The model under review builds one solid part; all positions refer to its coordinate system, in mm. A direction names the side the tool comes from. Give positions to 0.01 mm unless a question says otherwise; leave off trailing zeros. Order: outer loops, then holes, each group sorted by start corner. A loop starts at its lowest first (then second) coordinate and runs counter-clockwise, first axis right, second up.
```python
from build123d import *

# Parameters (mm, degrees)
F1_DEPTH      = 20
F2_DEPTH      = 15
F4_W          = 3.3256819006
F4_H          = 11.2064601853
F5_DEPTH      = 5.2
F5_DEPTH_BACK = 20
F3_R          = 3.6353661433
F6_DEPTH      = 25
F7_T1_DEPTH   = 11.2064601853
F7_T3_DEPTH   = 3.3256819006
F7_T5_DEPTH   = 3.3256819006
F7_T11_DEPTH  = 8.3256819006
F7_T16_DEPTH  = 16.2064601853
F7_T23_DEPTH  = 16.2064601853
F7_T27_DEPTH  = 8.3256819006
F7_T35_DEPTH  = 8.3256819006
F7_T40_DEPTH  = 16.2064601853
F7_T47_DEPTH  = 16.2064601853
F7_T51_DEPTH  = 8.3256819006
F7_T55_DEPTH  = 21.2064601853


# Not quite as in the source:
# - a fillet or chamfer that OpenCascade refuses, or shapes differently, is made with other operations: its cross-section is extruded or revolved along the edge and cut away or added


with BuildPart() as f1:
    # F0 (on Front) → F1 (new body)
    with BuildSketch(Plane.XZ):
        Polygon((7.3840099636, 4.3827313822), (-0.1035517331, 8.5861059014), (-7.4875616967, 4.2033745192), (-7.3840099636, -4.3827313822), (0.1035517331, -8.5861059014), (7.4875616967, -4.2033745192), align=None)
        Polygon((-2.8867513459, 5), (2.8867513459, 5), (5.7735026919, 0), (2.8867513459, -5), (-2.8867513459, -5), (-5.7735026919, 0), align=None, mode=Mode.SUBTRACT)
    extrude(amount=F1_DEPTH)

    # F0 (on Front) → F2 (join)
    with BuildSketch(Plane.XZ):
        Polygon((5.7735026919, 0), (2.8867513459, 5), (-2.8867513459, 5), (-5.7735026919, 0), (-2.8867513459, -5), (2.8867513459, -5), align=None)
    extrude(amount=F2_DEPTH)

    # F4 (on face) → F5 (join, two sides)
    with BuildSketch(Plane(origin=(-3.7955567149, 0, 6.3947402103), x_dir=(0.8599326743, 0, 0.51040748), z_dir=(-0.51040748, 0, 0.8599326743))) as f5_sk:
        with Locations((0, -5.6032300927)):
            Rectangle(F4_W, F4_H)
    extrude(amount=F5_DEPTH)
    extrude(f5_sk.sketch, amount=-F5_DEPTH_BACK)

    # F3 (on face) → F6 (cut)
    with BuildSketch(Plane.XZ.offset(15)):
        Circle(F3_R)
    extrude(amount=-F6_DEPTH, mode=Mode.SUBTRACT)

    # F7: fillet of radius 2 on 10 edges, made by hand

    # F7_s2 → F7_t1 (join)
    with BuildSketch(Plane.XZ):
        with BuildLine():
            ThreePointArc((-6.9453533288, 4.525198791), (-6.0282146576, 5.7507608695), (-6.2463029403, 7.2658790997))
            Line((-6.2463029403, 7.2658790997), (-5.2254879802, 5.5460137511))
            Line((-5.2254879802, 5.5460137511), (-6.9453533288, 4.525198791))
        make_face()
        with BuildLine():
            ThreePointArc((-0.645760101, 8.2642816296), (-2.1608783312, 8.0461933468), (-3.3864404097, 8.963332018))
            Line((-3.3864404097, 8.963332018), (-2.3656254496, 7.2434666695))
            Line((-2.3656254496, 7.2434666695), (-0.645760101, 8.2642816296))
        make_face()
        with BuildLine():
            ThreePointArc((6.9453533288, -4.525198791), (6.0282146576, -5.7507608695), (6.2463029403, -7.2658790997))
            Line((6.2463029403, -7.2658790997), (5.2254879802, -5.5460137511))
            Line((5.2254879802, -5.5460137511), (6.9453533288, -4.525198791))
        make_face()
        with BuildLine():
            ThreePointArc((0.645760101, -8.2642816296), (2.1608783312, -8.0461933468), (3.3864404097, -8.963332018))
            Line((3.3864404097, -8.963332018), (2.3656254496, -7.2434666695))
            Line((2.3656254496, -7.2434666695), (0.645760101, -8.2642816296))
        make_face()
    extrude(amount=F7_T1_DEPTH)

    # F7_s4 → F7_t3 (join)
    with BuildSketch(Plane(origin=(-1.4299312653, 0, -0.8487264592), x_dir=(0, 1, 0), z_dir=(0.8599326743, 0, 0.51040748))):
        with BuildLine():
            ThreePointArc((-13.2064601853, 7.4363265887), (-11.792246623, 8.0221130263), (-11.2064601853, 9.4363265887))
            Line((-11.2064601853, 9.4363265887), (-11.2064601853, 7.4363265887))
            Line((-11.2064601853, 7.4363265887), (-13.2064601853, 7.4363265887))
        make_face()
    extrude(amount=F7_T3_DEPTH)

    # F7_s6 → F7_t5 (join)
    with BuildSketch(Plane(origin=(1.4299312653, 0, 0.8487264592), x_dir=(0, 1, 0), z_dir=(-0.8599326743, 0, -0.51040748))):
        with BuildLine():
            ThreePointArc((-13.2064601853, 7.4363265887), (-11.792246623, 8.0221130263), (-11.2064601853, 9.4363265887))
            Line((-11.2064601853, 9.4363265887), (-11.2064601853, 7.4363265887))
            Line((-11.2064601853, 7.4363265887), (-13.2064601853, 7.4363265887))
        make_face()
    extrude(amount=F7_T5_DEPTH)


with BuildPart() as f7_tool9:
    # F7_s10 → F7_t11 (new body)
    with BuildSketch(Plane(origin=(-5.7295946368, 0, -3.4007638594), x_dir=(0, 1, 0), z_dir=(0.8599326743, 0, 0.51040748))):
        with BuildLine():
            ThreePointArc((-13.2064601853, 7.4363265887), (-11.792246623, 8.0221130263), (-11.2064601853, 9.4363265887))
            Line((-11.2064601853, 9.4363265887), (-11.2064601853, 7.4363265887))
            Line((-11.2064601853, 7.4363265887), (-13.2064601853, 7.4363265887))
        make_face()
    extrude(amount=F7_T11_DEPTH)

    split(bisect_by=Plane(origin=(-7.4357858302, 0, -0.0896784315), x_dir=(0, 1, 0), z_dir=(0.9999272815, 0, 0.0120595069)), keep=Keep.TOP)

    split(bisect_by=Plane(origin=(-1.4299312653, 0, -0.8487264592), x_dir=(0, 1, 0), z_dir=(-0.8599326743, 0, -0.51040748)), keep=Keep.TOP)


with BuildPart() as f7_tool14:
    # F7_s15 → F7_t16 (new body)
    with BuildSketch(Plane.XZ):
        with BuildLine():
            ThreePointArc((-6.9453533288, 4.525198791), (-6.0282146576, 5.7507608695), (-6.2463029403, 7.2658790997))
            Line((-6.2463029403, 7.2658790997), (-5.2254879802, 5.5460137511))
            Line((-5.2254879802, 5.5460137511), (-6.9453533288, 4.525198791))
        make_face()
    extrude(amount=F7_T16_DEPTH)

    split(bisect_by=Plane.XZ.offset(11.2064601853), keep=Keep.TOP)


with BuildPart() as f7_tool9_1:
    add(f7_tool9.part)

    # F7_t18: intersect F7_tool14
    add(f7_tool14.part, mode=Mode.INTERSECT)


with BuildPart() as f1_1:
    add(f1.part)

    # F7_t7: union F7_tool9
    add(f7_tool9_1.part)


with BuildPart() as f7_tool21:
    # F7_s22 → F7_t23 (new body)
    with BuildSketch(Plane.XZ.offset(16.2064601853)):
        with BuildLine():
            ThreePointArc((-0.645760101, 8.2642816296), (-2.1608783312, 8.0461933468), (-3.3864404097, 8.963332018))
            Line((-3.3864404097, 8.963332018), (-2.3656254496, 7.2434666695))
            Line((-2.3656254496, 7.2434666695), (-0.645760101, 8.2642816296))
        make_face()
    extrude(amount=-F7_T23_DEPTH)

    split(bisect_by=Plane.XZ.offset(11.2064601853), keep=Keep.TOP)


with BuildPart() as f7_tool25:
    # F7_s26 → F7_t27 (new body)
    with BuildSketch(Plane(origin=(-1.4299312653, 0, -0.8487264592), x_dir=(0, 1, 0), z_dir=(0.8599326743, 0, 0.51040748))):
        with BuildLine():
            ThreePointArc((-13.2064601853, 7.4363265887), (-11.792246623, 8.0221130263), (-11.2064601853, 9.4363265887))
            Line((-11.2064601853, 9.4363265887), (-11.2064601853, 7.4363265887))
            Line((-11.2064601853, 7.4363265887), (-13.2064601853, 7.4363265887))
        make_face()
    extrude(amount=F7_T27_DEPTH)

    split(bisect_by=Plane(origin=(3.6402291153, 0, 6.4844186418), x_dir=(0, 1, 0), z_dir=(-0.4895198015, 0, -0.8719921811)), keep=Keep.TOP)

    split(bisect_by=Plane(origin=(1.4299312653, 0, 0.8487264592), x_dir=(0, 1, 0), z_dir=(0.8599326743, 0, 0.51040748)), keep=Keep.TOP)


with BuildPart() as f7_tool21_1:
    add(f7_tool21.part)

    # F7_t30: intersect F7_tool25
    add(f7_tool25.part, mode=Mode.INTERSECT)


with BuildPart() as f1_2:
    add(f1_1.part)

    # F7_t19: union F7_tool21
    add(f7_tool21_1.part)


with BuildPart() as f7_tool33:
    # F7_s34 → F7_t35 (new body)
    with BuildSketch(Plane(origin=(5.7295946368, 0, 3.4007638594), x_dir=(0, 1, 0), z_dir=(-0.8599326743, 0, -0.51040748))):
        with BuildLine():
            ThreePointArc((-13.2064601853, 7.4363265887), (-11.792246623, 8.0221130263), (-11.2064601853, 9.4363265887))
            Line((-11.2064601853, 9.4363265887), (-11.2064601853, 7.4363265887))
            Line((-11.2064601853, 7.4363265887), (-13.2064601853, 7.4363265887))
        make_face()
    extrude(amount=F7_T35_DEPTH)

    split(bisect_by=Plane(origin=(7.4357858302, 0, 0.0896784315), x_dir=(0, 1, 0), z_dir=(-0.9999272815, 0, -0.0120595069)), keep=Keep.TOP)

    split(bisect_by=Plane(origin=(1.4299312653, 0, 0.8487264592), x_dir=(0, 1, 0), z_dir=(0.8599326743, 0, 0.51040748)), keep=Keep.TOP)


with BuildPart() as f7_tool38:
    # F7_s39 → F7_t40 (new body)
    with BuildSketch(Plane.XZ):
        with BuildLine():
            ThreePointArc((6.9453533288, -4.525198791), (6.0282146576, -5.7507608695), (6.2463029403, -7.2658790997))
            Line((6.2463029403, -7.2658790997), (5.2254879802, -5.5460137511))
            Line((5.2254879802, -5.5460137511), (6.9453533288, -4.525198791))
        make_face()
    extrude(amount=F7_T40_DEPTH)

    split(bisect_by=Plane.XZ.offset(11.2064601853), keep=Keep.TOP)


with BuildPart() as f7_tool33_1:
    add(f7_tool33.part)

    # F7_t42: intersect F7_tool38
    add(f7_tool38.part, mode=Mode.INTERSECT)


with BuildPart() as f1_3:
    add(f1_2.part)

    # F7_t31: union F7_tool33
    add(f7_tool33_1.part)


with BuildPart() as f7_tool45:
    # F7_s46 → F7_t47 (new body)
    with BuildSketch(Plane.XZ.offset(16.2064601853)):
        with BuildLine():
            ThreePointArc((0.645760101, -8.2642816296), (2.1608783312, -8.0461933468), (3.3864404097, -8.963332018))
            Line((3.3864404097, -8.963332018), (2.3656254496, -7.2434666695))
            Line((2.3656254496, -7.2434666695), (0.645760101, -8.2642816296))
        make_face()
    extrude(amount=-F7_T47_DEPTH)

    split(bisect_by=Plane.XZ.offset(11.2064601853), keep=Keep.TOP)


with BuildPart() as f7_tool49:
    # F7_s50 → F7_t51 (new body)
    with BuildSketch(Plane(origin=(1.4299312653, 0, 0.8487264592), x_dir=(0, 1, 0), z_dir=(-0.8599326743, 0, -0.51040748))):
        with BuildLine():
            ThreePointArc((-13.2064601853, 7.4363265887), (-11.792246623, 8.0221130263), (-11.2064601853, 9.4363265887))
            Line((-11.2064601853, 9.4363265887), (-11.2064601853, 7.4363265887))
            Line((-11.2064601853, 7.4363265887), (-13.2064601853, 7.4363265887))
        make_face()
    extrude(amount=F7_T51_DEPTH)

    split(bisect_by=Plane(origin=(-3.6402291153, 0, -6.4844186418), x_dir=(0, 1, 0), z_dir=(0.4895198015, 0, 0.8719921811)), keep=Keep.TOP)

    split(bisect_by=Plane(origin=(-1.4299312653, 0, -0.8487264592), x_dir=(0, 1, 0), z_dir=(-0.8599326743, 0, -0.51040748)), keep=Keep.TOP)


with BuildPart() as f7_tool45_1:
    add(f7_tool45.part)

    # F7_t54: intersect F7_tool49
    add(f7_tool49.part, mode=Mode.INTERSECT)


with BuildPart() as f1_4:
    add(f1_3.part)

    # F7_t43: union F7_tool45
    add(f7_tool45_1.part)

    # F7_s56 → F7_t55 (cut)
    with BuildSketch(Plane.XZ.offset(-5)):
        with BuildLine():
            ThreePointArc((-6.1597415279, 11.0384786175), (-7.0768801991, 9.8129165391), (-6.8587919164, 8.2977983089))
            Line((-6.8587919164, 8.2977983089), (-7.8796068765, 10.0176636575))
            Line((-7.8796068765, 10.0176636575), (-6.1597415279, 11.0384786175))
        make_face()
        with BuildLine():
            ThreePointArc((-3.9989293858, 9.9952512272), (-5.2244914642, 10.9123898984), (-6.7396096944, 10.6943016157))
            Line((-6.7396096944, 10.6943016157), (-5.0197443458, 11.7151165758))
            Line((-5.0197443458, 11.7151165758), (-3.9989293858, 9.9952512272))
        make_face()
        with BuildLine():
            ThreePointArc((6.7025269693, -10.6318247746), (5.1874087391, -10.8499130573), (3.9618466606, -9.9327743861))
            Line((3.9618466606, -9.9327743861), (4.9826616207, -11.6526397347))
            Line((4.9826616207, -11.6526397347), (6.7025269693, -10.6318247746))
        make_face()
        with BuildLine():
            ThreePointArc((6.8217091912, -8.2353214678), (7.039797474, -9.750439698), (6.1226588027, -10.9760017765))
            Line((6.1226588027, -10.9760017765), (7.8425241513, -9.9551868164))
            Line((7.8425241513, -9.9551868164), (6.8217091912, -8.2353214678))
        make_face()
    extrude(amount=F7_T55_DEPTH, mode=Mode.SUBTRACT)


solid = f1_4.part
```
Item 1: Draft analysis for pull direction X (two halves, no side actions). For faces 1 (the cylindrical face through (4.018, -12.077, -6.669)), 2 (the cylindrical face through (-2.14, -6.7, 8.04)), 3 (the cylindrical face through (-6.034, -6.511, 5.729)), state which applies: released by +X, released by -X, zero draft, split by the parting line, or undercut.
Values found:
face 1: released by +X
face 2: undercut
face 3: released by -X
Item 2: Take a section at A-A (y = -18.5). Give the boundary of the cut face in (x, z), and give its area (3 significant figures).
Values found:
outline: (-7.49, 4.2) - (-7.38, -4.38) - (0.1, -8.59) - (7.49, -4.2) - (7.38, 4.38) - (-0.1, 8.59) - close; hole (-5.77, 0) - (-2.89, -5) - (2.89, -5) - (5.77, 0) - (2.89, 5) - (-2.89, 5) - close
area: 105 mm2
Item 3: Clearance check with flat-ended pins moving along their axes: pin 1 Ø2.5 at (x, y) = (0.5, -16.5) entering from +Z; pin 2 Ø1.5 at (x, y) = (-5, -10.5) entering from -Z; pin 3 Ø1.8 at (x, z) = (5.5, -9.5) entering from -Y. State where each tip first meets the part, or that it passes through.
Values found:
pin 1: stops at z = 8.59
pin 2: stops at z = -6.14
pin 3: stops at y = -11.21
Item 4: For line 1 (Z direction, x = 2, y = -8.25); line 2 (Z direction, x = 1.5, y = -14.75); line 3 (X direction, y = -9.75, z = -1), list the stretches that pass through material, from the lowest coordinate up.
Values found:
line 1: z = -8.01 to -3.04, 3.04 to 7.41
line 2: z = -7.76 to -3.31, 3.31 to 7.69
line 3: x = -7.42 to -3.5, 3.5 to 7.45
Item 5: For faces 4 (the flat face through (-6.548, -5.682, 7.775)), 5 (the flat face through (-3.74, -14.3, 6.43)), 6 (the flat face through (6.53, -5.68, -7.74)), list the 3-axis set-ups (+Z, -Z, +X, -X, +Y, -Y) from which the entire face can be reached by the end or side of a thin tool; tool diameter is ignored.
Values found:
face 4: -X, +Y, -Y
face 5: -Y
face 6: +X, +Y, -Y
Item 6: Take a section at B-B (y = -6.5). Give the boundary of the cut face in (x, z), and give its area (3 significant figures).
Values found:
outline: (-7.49, 4.2) - (-7.38, -4.38) - (0.1, -8.59) - (0.65, -8.26) arc R2 cw to (3.39, -8.96) - (3.96, -9.93) arc R2 ccw to (6.4, -10.78) arc R2 ccw to (6.82, -8.24) - (6.25, -7.27) arc R2 cw to (6.95, -4.53) - (7.49, -4.2) - (7.38, 4.38) - (-0.1, 8.59) - (-0.65, 8.26) arc R2 cw to (-3.39, 8.96) - (-4, 10) arc R2 ccw to (-6.44, 10.84) arc R2 ccw to (-6.86, 8.3) - (-6.25, 7.27) arc R2 cw to (-6.95, 4.53) - close; hole circle Ø7.27 at (0, 0)
area: 184 mm2
